```python
from build123d import *

# Parameters (mm, degrees)
BOSS_EXTRUDE1_DEPTH    = 9.525
CUT_EXTRUDE1_DEPTH     = 239.991257685
CUT_EXTRUDE3_DEPTH     = 239.991257685
F_10_CLEARANCE_HOLE1_D = 5.1054
FILLET1_R              = 9.525
FILLET2_R              = 12.7
CUT_EXTRUDE4_DEPTH     = 239.991257685
FILLET3_R              = 0.79375


with BuildPart() as part:
    # Sketch1 → Boss-Extrude1 (new body)
    with BuildSketch(Plane(origin=(0, 0, 0), x_dir=(0, 0, -1), z_dir=(1, 0, 0))):
        Polygon((-193.675, 0), (193.675, 0), (193.675, 50.8), (54.76875, 50.8), (16.66875, 88.9), (16.66875, 139.7), (-16.66875, 139.7), (-16.66875, 88.9), (-54.76875, 50.8), (-193.675, 50.8), align=None)
    extrude(amount=BOSS_EXTRUDE1_DEPTH)

    # Sketch2 → Cut-Extrude1 (cut, through all)
    with BuildSketch(Plane(origin=(9.525, 0, 0), x_dir=(0, 0, -1), z_dir=(1, 0, 0))):
        with BuildLine():
            Line((-184.15, 34.528125), (-57.15, 34.528125))
            ThreePointArc((-57.15, 34.528125), (-53.578125, 38.1), (-57.15, 41.671875))
            Line((-57.15, 41.671875), (-184.15, 41.671875))
            ThreePointArc((-184.15, 41.671875), (-187.721875, 38.1), (-184.15, 34.528125))
        make_face()
        with BuildLine():
            Line((-184.15, 15.478125), (-57.15, 15.478125))
            ThreePointArc((-57.15, 15.478125), (-53.578125, 19.05), (-57.15, 22.621875))
            Line((-57.15, 22.621875), (-184.15, 22.621875))
            ThreePointArc((-184.15, 22.621875), (-187.721875, 19.05), (-184.15, 15.478125))
        make_face()
    cut_extrude1 = extrude(amount=-CUT_EXTRUDE1_DEPTH, mode=Mode.SUBTRACT)

    # Mirror1: Cut-Extrude1 across plane
    add(cut_extrude1.mirror(Plane.XY), mode=Mode.SUBTRACT)

    # Sketch4 → Cut-Extrude3 (cut, through all)
    with BuildSketch(Plane(origin=(9.525, 0, 0), x_dir=(0, 0, -1), z_dir=(1, 0, 0))):
        Polygon((-51.687213274, 0), (-19.937213274, 31.75), (19.937213274, 31.75), (51.687213274, 0), align=None)
    extrude(amount=-CUT_EXTRUDE3_DEPTH, mode=Mode.SUBTRACT)

    # #10 Clearance Hole1 (through all)
    with Locations(Plane(origin=(9.525, 0, 0), x_dir=(0, 0, -1), z_dir=(1, 0, 0))):
        with Locations((-11.90625, 127), (11.90625, 127), (-11.90625, 114.3), (-11.90625, 38.1), (11.90625, 114.3), (-11.90625, 50.8)):
            Hole(F_10_CLEARANCE_HOLE1_D / 2)

    # Fillet1
    fillet1_edges = [part.edges().sort_by_distance(p)[0] for p in [
        (4.7625, 139.7, 16.66875),
        (4.7625, 139.7, -16.66875),
    ]]
    fillet(fillet1_edges, radius=FILLET1_R)

    # Fillet2
    fillet2_edges = [part.edges().sort_by_distance(p)[0] for p in [
        (4.7625, 50.8, 193.675),
        (4.7625, 50.8, 54.76875),
        (4.7625, 88.9, 16.66875),
        (4.7625, 88.9, -16.66875),
        (4.7625, 50.8, -54.76875),
        (4.7625, 50.8, -193.675),
        (4.7625, 0, -193.675),
        (4.7625, 0, 193.675),
        (4.7625, 31.75, 19.937213274),
        (4.7625, 31.75, -19.937213274),
        (4.7625, 0, -51.687213274),
        (4.7625, 0, 51.687213274),
    ]]
    fillet(fillet2_edges, radius=FILLET2_R)

    # Sketch7 → Cut-Extrude4 (cut, through all)
    with BuildSketch(Plane(origin=(9.525, 0, 0), x_dir=(0, 0, -1), z_dir=(1, 0, 0))):
        with BuildLine():
            Line((11.90625, 129.5527), (16.66875, 129.5527))
            ThreePointArc((16.66875, 129.5527), (19.22145, 127), (16.66875, 124.4473))
            Line((16.66875, 124.4473), (11.90625, 124.4473))
            Line((11.90625, 124.4473), (8.73125, 124.4473))
            ThreePointArc((8.73125, 124.4473), (6.17855, 127), (8.73125, 129.5527))
            Line((8.73125, 129.5527), (11.90625, 129.5527))
        make_face()
        with BuildLine():
            Line((16.66875, 116.8527), (11.90625, 116.8527))
            Line((11.90625, 116.8527), (8.73125, 116.8527))
            ThreePointArc((8.73125, 116.8527), (6.17855, 114.3), (8.73125, 111.7473))
            Line((8.73125, 111.7473), (11.90625, 111.7473))
            Line((11.90625, 111.7473), (16.66875, 111.7473))
            ThreePointArc((16.66875, 111.7473), (19.22145, 114.3), (16.66875, 116.8527))
        make_face()
    extrude(amount=-CUT_EXTRUDE4_DEPTH, mode=Mode.SUBTRACT)

    # Fillet3
    fillet3_edges = [part.edges().sort_by_distance(p)[0] for p in [
        (4.7625, 111.7473, -16.66875),
        (4.7625, 116.8527, -16.66875),
        (4.7625, 124.4473, -16.66875),
        (4.7625, 129.5527, -16.66875),
    ]]
    fillet(fillet3_edges, radius=FILLET3_R)


solid = part.part
```
Verification items for the finished model (mm, model axes). A direction names the side the tool comes from. Round coordinates to 2 decimals unless told otherwise and drop trailing zeros. Write each loop counter-clockwise with the first axis right and the second up, starting at its lowest first coordinate (ties: lowest second). Pieces come first, ordered by that corner, then holes. Notation, with made-up numbers: (-18.75, -8) -> (34.25, -8) arc R23 cw to (34.25, 1) -> close; hole circle Ø9 at (65.5, -19). An arc over 180 degrees is marked (long way). Write each question's results on one line, items separated by ' | '. Start each with the question number.
1. Cross-section at C-C (z = -41.5). Enter the section's corners in (x, y) (3 decimals).
2. Set-up check for faces 1 (the cylindrical face through (4.83, 136.84, 13.95)), 2 (the flat face through (0, 39, 1)), 3 (the flat face through (5, 116.853, -12)), 4 (the cylindrical face through (4.83, 38.02, -53.58)), 5 (the cylindrical face through (4.7, 0.94, 52.15)): record each of +Z, -Z, +X, -X, +Y, -Y from which the full face is reachable in a straight line by a thin tool's end or side.
3. Draft check along Y on faces 6 (the cylindrical face through (4.829, 51.794, 55.105)), 7 (the flat face through (5, 22.622, 120)), 8 (the flat face through (5, 15.478, -122)), 9 (the flat face through (5, 102, -16.669)). Enter one of: +Y half, -Y half, draft (parallel to the pull), parting line (faces both ways), or undercut.
4. Cross-section at D-D (y = 70). Enter the section's corners in (x, z) (3 decimals).
5. Material ranges on probe 1 along Y at (x, z) = (3.5, -102.5); probe 2 along Y at (x, z) = (7.75, 56); probe 3 along Y at (x, z) = (3.5, -4), recorded low to high. Write a range as from..to.
6. Cross-section at B-B (x = 7.5). Count the separate pieces of the cut face and the enclosed holes in it, then the cut area to 3 significant figures.
7. Cross-section at A-A (y = 19.05). Enter the section's corners in (x, z) (3 decimals).
8. Depth check by flat-ended pin: P1, Ø2, axis at x = 6, z = -11.5, coming from the -Y side; P2, Ø1.8, axis at x = 3, y = 120, coming from the -Z side; P3, Ø2, axis at x = 5, z = 77.5, coming from the +Y side. Enter the tip coordinate at first touch or a pass-through.
Solutions:
1) outline: (0, 10.187) -> (9.525, 10.187) -> (9.525, 64.069) -> (0, 64.069) -> close
2) face 1: +Z, +X, -X, +Y | face 2: +Z, -Z, -X, +Y, -Y | face 3: -Z, +X, -X | face 4: +X, -X | face 5: +X, -X, -Y
3) face 6: +Y half | face 7: undercut | face 8: undercut | face 9: draft
4) outline: (0, -35.569) -> (9.525, -35.569) -> (9.525, 35.569) -> (0, 35.569) -> close
5) probe 1: y = 0..15.48, 22.62..34.53, 41.67..50.8 | probe 2: y = 0.04..15.67, 22.43..34.72, 41.48..51.46 | probe 3: y = 31.75..139.7
6) separate pieces: 1 | enclosed holes: 8 | area: 17,700 mm2
7) outline: (0, -193.675) -> (9.525, -193.675) -> (9.525, -187.722) -> (0, -187.722) -> close; (0, -53.578) -> (9.525, -53.578) -> (9.525, -32.637) -> (0, -32.637) -> close; (0, 32.637) -> (9.525, 32.637) -> (9.525, 53.578) -> (0, 53.578) -> close; (0, 187.722) -> (9.525, 187.722) -> (9.525, 193.675) -> (0, 193.675) -> close
8) P1: stops at y = 31.75 | P2: stops at z = -16.67 | P3: stops at y = 50.8
